Autodesk Inventor part; units mm, degrees
ref_plane "YZ Plane" through (0, 0, 0) normal (1, 0, 0) x (0, 1, 0)
ref_plane "XZ Plane" through (0, 0, 0) normal (0, 1, 0) x (-1, 0, 0)
ref_plane "XY Plane" through (0, 0, 0) normal (0, 0, 1) x (1, 0, 0)
sketch "Sketch_40" plane through (0, 0, 0) normal (0, 0, 1) x (1, 0, 0)
  line L0 (2.5, 0) -> (-2.5, 0)
  line L1 (0, 5.2) -> (0, 4.2)
  arc A0 (0, 4.2) -> (0.2, 4) centre (0.2, 4.2) ccw
  line L2 (0.2, 4) -> (4.8, 4)
  arc A1 (4.8, 4) -> (5, 4.2) centre (4.8, 4.2) ccw
  line L3 (5, 4.2) -> (5, 5.2)
  arc A2 (5, 5.2) -> (4.95, 5.25) centre (4.95, 5.2) ccw
  line L4 (4.95, 5.25) -> (3.1614, 5.25)
  arc A3 (1.8386, 5.25) -> (3.1614, 5.25) centre (2.5, 6) ccw
  line L5 (1.8386, 5.25) -> (0.05, 5.25)
  arc A4 (0.05, 5.25) -> (0, 5.2) centre (0.05, 5.2) ccw
revolve "Revolution1" add sketch "Sketch_40" angle 360 about axis through (2.5, 0, 0) along (1, 0, 0)
sketch "Sketch_42" plane through (0, 0, 0) normal (0, 0, 1) x (1, 0, 0)
  line L0 (2.5, 0) -> (-2.5, 0)
  line L1 (0, 10.825) -> (0, 4.825)
  line L2 (0, 4.825) -> (0.1, 4.825)
  arc A0 (0.1, 4.825) -> (0.3, 5.025) centre (0.1, 5.025) ccw
  line L3 (0.3, 5.025) -> (0.3, 10.625)
  line L4 (0.3, 10.625) -> (4.7, 10.625)
  line L5 (4.7, 10.625) -> (4.7, 5.025)
  arc A1 (4.7, 5.025) -> (4.9, 4.825) centre (4.9, 5.025) ccw
  line L6 (4.9, 4.825) -> (5, 4.825)
  line L7 (5, 4.825) -> (5, 10.825)
  line L8 (5, 10.825) -> (0, 10.825)
revolve "Revolution2" cut sketch "Sketch_42" angle 360 about axis through (2.5, 0, 0) along (1, 0, 0)
sketch "Sketch_44" plane through (0, 0, 0) normal (0, 0, 1) x (1, 0, 0)
  line L0 (5, 0) -> (-5, 0)
  line L1 (4.83, 5.2875) -> (4.89, 4.825)
  line L2 (4.89, 4.825) -> (4.95, 4.825)
  line L3 (4.95, 4.825) -> (4.92, 5.2875)
  line L4 (4.92, 5.2875) -> (4.95, 5.75)
  line L5 (4.95, 5.75) -> (4.95, 7.1)
  line L6 (4.95, 7.1) -> (4.9176, 7.1)
  line L7 (4.9176, 7.1) -> (4.83, 5.75)
  line L8 (4.83, 5.75) -> (4.83, 5.2875)
revolve "Revolution3" add sketch "Sketch_44" angle 360 about axis through (5, 0, 0) along (1, 0, 0)
sketch "Sketch_49" plane through (0, 0, 0) normal (0, 0, 1) x (1, 0, 0)
  line L0 (5, 0) -> (-5, 0)
  line L1 (0.07, 4.825) -> (0.13, 4.825)
  line L2 (0.13, 4.825) -> (0.19, 5.2875)
  line L3 (0.19, 5.2875) -> (0.19, 5.75)
  line L4 (0.19, 5.75) -> (0.1024, 7.1)
  line L5 (0.1024, 7.1) -> (0.07, 7.1)
  line L6 (0.07, 7.1) -> (0.07, 5.75)
  line L7 (0.07, 5.75) -> (0.1, 5.2875)
  line L8 (0.1, 5.2875) -> (0.07, 4.825)
revolve "Revolution4" add sketch "Sketch_49" angle 360 about axis through (5, 0, 0) along (1, 0, 0)
properties part number "SKF_W 628/8 R-2RS1_PART1"
Geometry: final body of the model. Coordinates: model frame, mm. Give positions to 0.01 mm unless a question says otherwise; leave off trailing zeros. Write each loop counter-clockwise with the first axis right and the second up, starting at its lowest first coordinate (ties: lowest second). Pieces come first, ordered by that corner, then holes. Notation, with made-up numbers: M 81,70 L 140,70 A38 ccw 140,109 Z; hole C 77.5,36.5 d7. An arc over 180 degrees is marked long. Answer in a Markdown table with one row per item. Add a question column.
(1) Mould query, pull axis Y, two halves, no side actions, for faces 1 (the cylindrical face through (2.532, -0.867, -3.905)), 2 (the cylindrical face through (1.1, 5, -1.6)), 3 (the flat face through (5, 2, 4)). Classes: +Y half, -Y half, draft (parallel to the pull), parting line (faces both ways), or undercut.
(2) Ray query, line 1 (Z direction, x = 1.4, y = 0); line 2 (Z direction, x = 2.9, y = 0); line 3 (Y direction, x = 1.6, z = -3). Return the intervals inside material, ascending.
(3) Section B-B on x = 4.45. Return loops of the section in (y, z), and give its area (3 significant figures).
(4) First-contact query: pin 1 (3 mm diameter, centred on x = 4, y = 4.5, fed in from +Z); pin 2 (1.5 mm diameter, centred on x = 4, y = -4.5, fed in from -Z); pin 3 (3 mm diameter, centred on x = 2, y = -2.5, fed in from -Z). Flat tips, straight axial feed; report the tip coordinate or a pass-through.
(5) Section A-A on x = 2.6. Return loops of the section in (y, z).
Result set:
| question | item | result |
|---|---|---|
| 1 | face 1 | undercut |
| 1 | face 2 | parting line |
| 1 | face 3 | draft |
| 2 | line 1 | z = -5.25 to -4, 4 to 5.25 |
| 2 | line 2 | z = -5.08 to -4, 4 to 5.08 |
| 2 | line 3 | y = -4.31 to -2.65, 2.65 to 4.31 |
| 3 | outline | C 0,0 d10.5; hole C 0,0 d8 |
| 3 | area | 36.3 mm^2 |
| 4 | pin 1 | stops at z = 6.28 |
| 4 | pin 2 | stops at z = -3.67 |
| 4 | pin 3 | stops at z = -5.15 |
| 5 | outline | C 0,0 d10.01; hole C 0,0 d8 |
